```python
from build123d import *

# Parameters (mm, degrees)
F0_W     = 50.8
F0_H     = 16.51
F3_DEPTH = 50.8
F6_DEPTH = 6.35
F4_W     = 11.2776
F4_H     = 8.89
F7_DEPTH = 6.35


with BuildPart() as f1:
    # F0 (on Front) → F1 (revolve)
    with BuildSketch(Plane.XZ):
        with Locations((-57.8927400278, 71.4143859753)):
            Rectangle(F0_W, F0_H)
    revolve(axis=Axis((-60.0075013936, 0, -38.4406140247), (1, 0, 0)))

    # F2 (on face) → F3 (join)
    with BuildSketch(Plane.YZ.offset(-32.4927400278)):
        with BuildLine():
            ThreePointArc((-41.8872153091, 71.992321704), (0.7051217623, 79.667281153), (43.2027846909, 71.484321704))
            Line((43.2027846909, 71.484321704), (43.2027846909, 91.042321704))
            Line((43.2027846909, 91.042321704), (-41.8872153091, 91.042321704))
            Line((-41.8872153091, 91.042321704), (-41.8872153091, 71.992321704))
        make_face()
    extrude(amount=-F3_DEPTH)

    # F5 (on face) → F6 (join)
    with BuildSketch(Plane.XY.offset(91.042321704)):
        Polygon((-38.3323021233, 17.4853205681), (-76.9100263715, 17.3771120608), (-76.9100263715, -41.4511188865), (-63.3748918772, -41.4511188865), (-63.3748918772, -7.5572687201), (-51.7171360552, -7.5572687201), (-51.7171360552, -41.4511188865), (-38.3323021233, -41.4511188865), align=None)
    extrude(amount=F6_DEPTH)

    # F4 (on face) → F7 (cut)
    with BuildSketch(Plane.XY.offset(91.042321704)):
        with Locations((-58.3582898628, 4.445)):
            Rectangle(F4_W, F4_H)
    extrude(amount=F7_DEPTH, mode=Mode.SUBTRACT)


solid = f1.part
```
Could you check a few things on this model? Use its own coordinates, in mm. A direction names the side the tool comes from. Give positions to 0.01 mm unless a question says otherwise; leave off trailing zeros. Order: outer loops, then holes, each group sorted by start corner. A loop starts at its lowest first (then second) coordinate and runs counter-clockwise, first axis right, second up.
Q1. I'm going to push flat-ended pins straight in: P1, Ø2.5, axis at x = -59.5, y = 6, coming from the +Z side; P2, Ø7, axis at x = -70.5, z = 96, coming from the -Y side; P3, Ø15.5, axis at x = -70.5, z = 79.5, coming from the +Y side. Where does each tip first touch, or does it pass through?
Q2. We'd pull the mould along Y, two halves only. Please class faces 1 (the flat face through (-76.91, -12, 94)), 2 (the flat face through (-58, 5, 91.042)), 3 (the flat face through (-70, -41.451, 94)): +Y half, -Y half, draft (parallel to the pull), parting line (faces both ways), or undercut.
Q3. Suppose I cut it at A-A, the plane y = 59.5. Write out the boundary of the cut face in (x, z).
Q4. If I drill on line 1 along Z through (x, y) = (-66, 0); line 2 along Y through (x, z) = (-45, -77); line 3 along Y through (x, z) = (-37, 0), over which ranges is the centre line in solid material (lowest first)?
Q5. Suppose I cut it at D-D, the plane x = -45.5. Write out the boundary of the cut face in (y, z).
Q6. Suppose I cut it at B-B, the plane z = -36.5. Write out the boundary of the cut face in (x, y).
Q7. Suppose I cut it at C-C, the plane x = -80. Write out the boundary of the cut face in (y, z), and give its area (3 significant figures).
Q8. For faces 4 (the cylindrical face through (-57.537, -4.467, -139.942)), 5 (the flat face through (-38.332, -12, 94)), 6 (the flat face through (-63.997, 4, 94)), 7 (the flat face through (-51.717, -24, 94)), 8 (the flat face through (-45, -41.451, 94)), which set-ups out of +Z, -Z, +X, -X, +Y, -Y let a thin tool reach every point of the face, with its end or its side?
Solution:
1. P1: stops at z = 91.04
1. P2: stops at y = -41.45
1. P3: stops at y = 43.2
2. face 1: draft
2. face 2: undercut
2. face 3: -Y half
3. outline: (-83.29, -140.47) - (-32.49, -140.47) - (-32.49, -120.8) - (-83.29, -120.8) - close; (-83.29, 43.91) - (-32.49, 43.91) - (-32.49, 63.59) - (-83.29, 63.59) - close
4. line 1: z = -156.55 to -140.04, 63.16 to 97.39
4. line 2: y = -111.64 to -94, 94 to 111.64
4. line 3: y = -111.68 to -94.05, 94.05 to 111.68
5. outline: (-41.89, 71.99) arc R118.11 ccw (long way) to (43.2, 71.48) - (43.2, 91.04) - (17.47, 91.04) - (17.47, 97.39) - (-41.45, 97.39) - (-41.45, 91.04) - (-41.89, 91.04) - close; hole circle Ø203.2 at (0, -38.44)
6. outline: (-83.29, -118.09) - (-32.49, -118.09) - (-32.49, -101.58) - (-83.29, -101.58) - close; (-83.29, 101.58) - (-32.49, 101.58) - (-32.49, 118.09) - (-83.29, 118.09) - close
7. outline: (-41.89, 71.99) arc R118.11 ccw (long way) to (43.2, 71.48) - (43.2, 91.04) - (-41.89, 91.04) - close; hole circle Ø203.2 at (0, -38.44)
7. area: 12,600 mm2
8. face 4: +X, -X
8. face 5: +Z, +X, +Y, -Y
8. face 6: +Z
8. face 7: +Z, -Y
8. face 8: +Z, +X, -X, -Y
